For this review, take the finished solid that the model builds, in its own axes (mm). A direction names the side the tool comes from. Coordinates: 2 decimals unless noted, no trailing zeros. Order: outer loops, then holes, each group sorted by start corner. A loop starts at its lowest first (then second) coordinate and runs counter-clockwise, first axis right, second up. Notation, with made-up numbers: (-28, -29) - (-10, -29) arc R26 cw to (-10, -2) - close; hole circle Ø1 at (-28.5, 12). An arc over 180 degrees is marked (long way). One line per item, written item: value. Start each with the question number.
(1) Mouldability with a two-part tool opening along Z and no side actions: class faces 6 (the flat face through (34, 10, 0)), 7 (the flat face through (34, 21, 8)), 8 (the flat face through (69.85, -1, -29)), 9 (the cylindrical face through (31.74, 21.22, 5.72)) as released by +Z, released by -Z, zero draft, split by the parting line, or undercut.
(2) Consider section D-D on z = -16. Write out the cut boundary in (x, y).
(3) Clearance check with flat-ended pins moving along their axes: pin 1 (7 mm diameter, centred on x = 16, y = 9, fed in from -Z); pin 2 (10 mm diameter, centred on y = 12.5, z = -40.5, fed in from +X); pin 3 (5.5 mm diameter, centred on x = 41.5, z = 6, fed in from -Y). State where each tip first meets the part, or that it passes through.
(4) For faces 1 (the flat face through (34, 8, 3)), 2 (the flat face through (0.5, 21.2, -70)), 3 (the flat face through (34, 8, -67.5)), 4 (the flat face through (0, 10, -33)), 5 (the flat face through (34, -3, -33)), list the 3-axis set-ups (+Z, -Z, +X, -X, +Y, -Y) from which the entire face can be reached by the end or side of a thin tool; tool diameter is ignored.
(5) To check wall thickness, follow line 1 along Y through (x, z) = (50, -22.5); line 2 along Z through (x, y) = (51.5, 14); line 3 along X through (y, z) = (18.75, -31). State the ranges of each line that lie inside material, in increasing order.
(6) Consider section A-A on x = 28.5. Write out the cut boundary in (y, z), then the cut area to 3 significant figures.
(7) Consider section B-B on z = -70. Write out the cut boundary in (x, y) (3 decimals).
(8) Consider section C-C on y = 17.25. Write out the cut boundary in (x, z), then the cut area to 3 significant figures.
```python
from build123d import *

# Parameters (mm, degrees)
SKETCH2_W           = 70.5
SKETCH2_H           = 25.7
SKETCH2_W_2         = 64.5
SKETCH2_H_2         = 19.7
BOSS_EXTRUDE1_DEPTH = 69.85
SKETCH3_W           = 70.5
SKETCH3_H           = 25.7
BOSS_EXTRUDE2_DEPTH = 3
SKETCH4_R           = 1.7
BOSS_EXTRUDE3_DEPTH = 3


with BuildPart() as part:
    # Sketch2 → Boss-Extrude1 (new body)
    with BuildSketch(Plane(origin=(0, 0, 0), x_dir=(0, 0, -1), z_dir=(1, 0, 0))):
        with Locations((32.25, 9.85)):
            Rectangle(SKETCH2_W, SKETCH2_H)
        with Locations((32.25, 9.85)):
            Rectangle(SKETCH2_W_2, SKETCH2_H_2, mode=Mode.SUBTRACT)
    extrude(amount=BOSS_EXTRUDE1_DEPTH)

    # Sketch3 → Boss-Extrude2 (add)
    with BuildSketch(Plane.ZY):
        with Locations((-32.25, 9.85)):
            Rectangle(SKETCH3_W, SKETCH3_H)
    extrude(amount=BOSS_EXTRUDE2_DEPTH)

    # Sketch4 → Boss-Extrude3 (add)
    # profile 1 of 2: a face of its own
    with BuildSketch(Plane(origin=(0, 22.7, 0), x_dir=(1, 0, 0), z_dir=(0, 1, 0))):
        Polygon((69.85, 67.5), (62.85, 72.5), (4, 72.5), (-3, 67.5), align=None)
        with Locations(Location((33.425, 70, 0), (0, 0, 270))):
            Circle(SKETCH4_R, mode=Mode.SUBTRACT)
    # profile 2 of 2: a face of its own
    with BuildSketch(Plane(origin=(0, 22.7, 0), x_dir=(1, 0, 0), z_dir=(0, 1, 0))):
        Polygon((-3, -3), (69.85, -3), (62.85, -8), (4, -8), align=None)
        with Locations(Location((33.425, -5.5, 0), (0, 0, 90))):
            Circle(SKETCH4_R, mode=Mode.SUBTRACT)
    extrude(amount=-BOSS_EXTRUDE3_DEPTH)


solid = part.part
```
Geometry check:
1. face 6: undercut
1. face 7: released by +Z
1. face 8: zero draft
1. face 9: undercut
2. outline: (-3, -3) - (69.85, -3) - (69.85, 0) - (0, 0) - (0, 19.7) - (69.85, 19.7) - (69.85, 22.7) - (-3, 22.7) - close
3. pin 1: stops at z = -67.5
3. pin 2: stops at x = 0
3. pin 3: stops at y = 19.7
4. face 1: +Z, +X, -X, -Y
4. face 2: -Z, -X, +Y, -Y
4. face 3: -Z, +X, -X, -Y
4. face 4: +X
4. face 5: +Z, -Z, +X, -X, -Y
5. line 1: y = -3 to 0, 19.7 to 22.7
5. line 2: z = -67.5 to -64.5, 0 to 3
5. line 3: x = -3 to 0
6. outline: (-3, -67.5) - (19.7, -67.5) - (19.7, -72.5) - (22.7, -72.5) - (22.7, 8) - (19.7, 8) - (19.7, 3) - (-3, 3) - close; hole (0, -64.5) - (19.7, -64.5) - (19.7, 0) - (0, 0) - close
6. area: 571 mm^2
7. outline: (0.5, 19.7) - (31.725, 19.7) - (31.725, 22.7) - (0.5, 22.7) - close; (35.125, 19.7) - (66.35, 19.7) - (66.35, 22.7) - (35.125, 22.7) - close
8. outline: (-3, -67.5) - (69.85, -67.5) - (69.85, -64.5) - (0, -64.5) - (0, 0) - (69.85, 0) - (69.85, 3) - (-3, 3) - close
8. area: 631 mm^2
